from build123d import *

# Parameters (mm, degrees)
PAD_DEPTH       = 50
SKETCH001_R     = 11.5
SKETCH001_R_2   = 1.8
POCKET_DEPTH    = 2.7
SKETCH002_R     = 2.4
POCKET001_DEPTH = 5


with BuildPart() as part:
    # Sketch → Pad (new body)
    with BuildSketch(Plane.XY):
        Polygon((-2.7, 2.7), (-53, 2.7), (-53, 0), (0, 0), (0, 52), (-2.7, 52), align=None)
    extrude(amount=PAD_DEPTH)

    # Sketch001 → Pocket (cut)
    with BuildSketch(Plane(origin=(-2.7, 0, 0), x_dir=(0, -1, 0), z_dir=(-1, 0, 0))):
        with Locations((-30.9, 25)):
            Circle(SKETCH001_R)
        with Locations((-46.4, 40.5)):
            Circle(SKETCH001_R_2)
        with Locations((-15.4, 40.5)):
            Circle(SKETCH001_R_2)
        with Locations((-15.4, 9.5)):
            Circle(SKETCH001_R_2)
        with Locations((-46.4, 9.5)):
            Circle(SKETCH001_R_2)
    extrude(amount=-POCKET_DEPTH, mode=Mode.SUBTRACT)

    # Sketch002 → Pocket001 (cut)
    with BuildSketch(Plane(origin=(0, 2.7, 0), x_dir=(-1, 0, 0), z_dir=(0, 1, 0))):
        with Locations((14, 39.9)):
            Circle(SKETCH002_R)
        with Locations((39, 39.9)):
            Circle(SKETCH002_R)
        with Locations((39, 10.1)):
            Circle(SKETCH002_R)
        with Locations((14, 10.1)):
            Circle(SKETCH002_R)
    extrude(amount=-POCKET001_DEPTH, mode=Mode.SUBTRACT)


solid = part.part
The model under review builds one solid part; all positions refer to its coordinate system, in mm. A direction names the side the tool comes from. Round coordinates to 2 decimals unless told otherwise and drop trailing zeros. Loops run counter-clockwise (first coordinate to the right, second up) from the corner with the lowest first, then second, coordinate; pieces in that order, holes last. Notation, with made-up numbers: (-26, 16.5) - (24, 16.5) arc R25 ccw to (24, 44.5) - close; hole circle Ø5 at (27, 84.25). An arc over 180 degrees is marked (long way). Use CSV: the item, a comma, the result in double quotes.
(1) For line 1 (Z direction, x = -39, y = 0.5); line 2 (X direction, y = 1, z = 10); line 3 (Z direction, x = -1.45, y = 15.4), list the stretches that pass through material, from the lowest coordinate up.
Working result:
line 1,"z = 0 to 7.7, 12.5 to 37.5, 42.3 to 50"
line 2,"x = -53 to -41.4, -36.6 to -16.4, -11.6 to 0"
line 3,"z = 0 to 7.7, 11.3 to 38.7, 42.3 to 50"
(2) Take a section at D-D, the plane y = 30.9. Give the boundary of the cut face in (x, z), plus the area to 3 significant figures.
Working result:
outline,"(-2.7, 0) - (0, 0) - (0, 13.5) - (-2.7, 13.5) - close; (-2.7, 36.5) - (0, 36.5) - (0, 50) - (-2.7, 50) - close"
area,"72.9 mm^2"
(3) Take a section at A-A, the plane y = 15.4. Give the boundary of the cut face in (x, z), plus the area to 3 significant figures.
Working result:
outline,"(-2.7, 0) - (0, 0) - (0, 7.7) - (-2.7, 7.7) - close; (-2.7, 11.3) - (0, 11.3) - (0, 38.7) - (-2.7, 38.7) - close; (-2.7, 42.3) - (0, 42.3) - (0, 50) - (-2.7, 50) - close"
area,"116 mm^2"
(4) Take a section at B-B, the plane x = -14. Give the boundary of the cut face in (y, z), plus the area to 3 significant figures.
Working result:
outline,"(0, 0) - (2.7, 0) - (2.7, 7.7) - (0, 7.7) - close; (0, 12.5) - (2.7, 12.5) - (2.7, 37.5) - (0, 37.5) - close; (0, 42.3) - (2.7, 42.3) - (2.7, 50) - (0, 50) - close"
area,"109 mm^2"
(5) The part is to be moulded in two halves that separate along Y. For faces 3 (the flat face through (-27, 0, 25)), 4 (the flat face through (0, 20, 19)), 5 (the flat face through (-27, 2.7, 25)), 6 (the cylindrical face through (-1.4, 32.4, 36.4)), say which applies: pulls with the +Y half, pulls with the -Y half, needs draft (parallel to the pull), parting line crosses it, or undercut.
Working result:
face 3,"pulls with the -Y half"
face 4,"needs draft"
face 5,"pulls with the +Y half"
face 6,"undercut"
(6) Machinability: for faces 1 (the flat face through (-2.7, 27.7, 13.5)), 2 (the cylindrical face through (-11.602, 1.369, 40.006)), which of the approach directions +Z, -Z, +X, -X, +Y, -Y give a long, thin tool a straight path to every point of the face, cutting with its end or side? Answer none if there is none.
Working result:
face 1,"+Z, -Z, -X, +Y"
face 2,"+Y, -Y"
(7) Clearance check with flat-ended pins moving along their axes: P1, Ø4, axis at x = -14, z = 39.9, coming from the +Y side; P2, Ø7.5, axis at x = -14, z = 10.1, coming from the +Y side; P3, Ø8, axis at x = -18, z = 14.5, coming from the -Y side. State where each tip first meets the part, or that it passes through.
Working result:
P1,"passes through"
P2,"stops at y = 2.7"
P3,"stops at y = 0"
(8) Take a section at C-C, the plane z = 16. Give the boundary of the cut face in (x, y), plus the area to 3 significant figures.
Working result:
outline,"(-53, 0) - (0, 0) - (0, 23.74) - (-2.7, 23.74) - (-2.7, 2.7) - (-53, 2.7) - close; (-2.7, 38.06) - (0, 38.06) - (0, 52) - (-2.7, 52) - close"
area,"238 mm^2"
